Verification items for the finished model (mm, model axes). A direction names the side the tool comes from. Round coordinates to 2 decimals unless told otherwise and drop trailing zeros. Order: outer loops, then holes, each group sorted by start corner. A loop starts at its lowest first (then second) coordinate and runs counter-clockwise, first axis right, second up. Notation, with made-up numbers: (-11, 87) -> (34, 87) arc R8 cw to (34, 98) -> close; hole circle Ø9 at (-14.5, 79.5). An arc over 180 degrees is marked (long way). Return JSON: item names as keys, results as strings. Group by question number.
1) Section check C-C on x = -30. Enter the section's corners in (y, z), plus the area to 3 significant figures.
2) Depth check by flat-ended pin: pin 1 (5.5 mm diameter, centred on y = -22.6, z = -110.5, fed in from -X); pin 2 (4 mm diameter, centred on y = -20.5, z = -120, fed in from -X); pin 3 (0.6 mm diameter, centred on y = -1.5, z = -167.5, fed in from -X); pin 4 (1.6 mm diameter, centred on y = -1, z = -167.5, fed in from +X). Enter the tip coordinate at first touch or a pass-through.
3) Section check B-B on z = -148.5. Enter the section's corners in (x, y), plus the area to 3 significant figures.
4) Section check A-A on z = -34.5. Enter the section's corners in (x, y).
5) Scan lines: L1, parallel to Y at x = -18, z = -66; L2, parallel to X at y = -1, z = -34. Record each from-to range of solid material in increasing order.
6) Tool access check on faces 4 (the flat face through (-11, -1, -177.8)), 5 (the flat face through (-2, -17.9, -87.7)), 6 (the cylindrical face through (-27.1, -1, -72.4)), 7 (the cylindrical face through (-1, -22.5, -160)). Record the directions out of +Z, -Z, +X, -X, +Y, -Y that give a thin tool (end or side, any length) a straight path to the whole face; none if there is none.
7) Draft check along X on faces 1 (the cylindrical face through (-27.1, -1, -148.4)), 2 (the flat face through (0, -17, -88)), 3 (the cylindrical face through (-1, -22.7, -175)). Enter one of: pulls with the +X half, pulls with the -X half, needs draft (parallel to the pull), parting line crosses it, or undercut.
```python
from build123d import *

# Parameters (mm, degrees)
STRUCTURAL_MEMBER1_DEPTH        = 177.8
SLOT_DEPTH                      = 187.62491795
SKETCH4_R                       = 4.5
HOLE_DEPTH                      = 187.62491795
VERT_SLOT_DEPTH                 = 187.62491795
SLOT_PATTERN_COUNT              = 5
SLOT_PATTERN_PITCH              = 38
HOLE_PATTERN_COUNT              = 2
HOLE_PATTERN_PITCH              = 76
LPATTERN1_COUNT                 = 2
LPATTERN1_PITCH                 = 76
OTHER_SIDE_CUTS_COUNT           = 2
OTHER_SIDE_CUTS_ANGLE           = 90
OTHER_SIDE_CUTS_COPY_1_DEPTH    = 187.62491795
OTHER_SIDE_CUTS_COPY_2_DEPTH    = 187.62491795
OTHER_SIDE_CUTS_COPY_3_DEPTH    = 187.62491795
OTHER_SIDE_CUTS_COPY_4_DEPTH    = 187.62491795
OTHER_SIDE_CUTS_COPY_5_SKETCH_R = 4.5
OTHER_SIDE_CUTS_COPY_5_DEPTH    = 187.62491795
OTHER_SIDE_CUTS_COPY_6_DEPTH    = 187.62491795


with BuildPart() as part:
    # Sketch13 → Structural Member1 (new body)
    with BuildSketch(Plane(origin=(0, 0, 0), x_dir=(-1, 0, 0), z_dir=(0, 0, -1))):
        with BuildLine():
            Line((40.1, 0), (2, 0))
            ThreePointArc((2, 0), (0.585786438, -0.585786438), (0, -2))
            Line((0, -2), (0, -40.1))
            Line((0, -40.1), (1, -40.1))
            ThreePointArc((1, -40.1), (1.707106781, -39.807106781), (2, -39.1))
            Line((2, -39.1), (2, -4))
            ThreePointArc((2, -4), (2.585786438, -2.585786438), (4, -2))
            Line((4, -2), (39.1, -2))
            ThreePointArc((39.1, -2), (39.807106781, -1.707106781), (40.1, -1))
            Line((40.1, -1), (40.1, 0))
        make_face()
    extrude(amount=STRUCTURAL_MEMBER1_DEPTH)

    # Sketch3 → Slot (cut, through all)
    with BuildSketch(Plane(origin=(0, 0, 0), x_dir=(1, 0, 0), z_dir=(0, 1, 0))):
        with BuildLine():
            Line((-27.1, 12.5), (-27.1, 18.5))
            ThreePointArc((-27.1, 18.5), (-22.6, 23), (-18.1, 18.5))
            Line((-18.1, 18.5), (-18.1, 12.5))
            ThreePointArc((-18.1, 12.5), (-22.6, 8), (-27.1, 12.5))
        make_face()
    slot = extrude(amount=-SLOT_DEPTH, mode=Mode.SUBTRACT)

    # Sketch4 → Hole (cut, through all)
    with BuildSketch(Plane(origin=(0, 0, 0), x_dir=(1, 0, 0), z_dir=(0, 1, 0))):
        with Locations(Location((-22.6, 34.5, 0), (0, 0, 180))):
            Circle(SKETCH4_R)
    hole = extrude(amount=-HOLE_DEPTH, mode=Mode.SUBTRACT)

    # Sketch14 → Vert Slot (cut, through all)
    with BuildSketch(Plane(origin=(0, 0, 0), x_dir=(1, 0, 0), z_dir=(0, 1, 0))):
        with BuildLine():
            Line((-19.6, 68), (-22.6, 68))
            ThreePointArc((-22.6, 68), (-27.1, 72.5), (-22.6, 77))
            Line((-22.6, 77), (-19.6, 77))
            ThreePointArc((-19.6, 77), (-15.1, 72.5), (-19.6, 68))
        make_face()
    vert_slot = extrude(amount=-VERT_SLOT_DEPTH, mode=Mode.SUBTRACT)

    # Slot Pattern: Slot ×5
    with Locations(*[(0, 0, -i * SLOT_PATTERN_PITCH) for i in range(1, SLOT_PATTERN_COUNT)]):
        add(slot, mode=Mode.SUBTRACT)

    # Hole Pattern: Hole ×2
    with Locations(*[(0, 0, -i * HOLE_PATTERN_PITCH) for i in range(1, HOLE_PATTERN_COUNT)]):
        add(hole, mode=Mode.SUBTRACT)

    # LPattern1: Vert Slot ×2
    with Locations(*[(0, 0, -i * LPATTERN1_PITCH) for i in range(1, LPATTERN1_COUNT)]):
        add(vert_slot, mode=Mode.SUBTRACT)

    # Other side cuts: Slot, Hole, Vert Slot ×2 about axis
    other_side_cuts_axis = Axis((-4, -4, 0), (0, 0, 1))
    add([slot.rotate(other_side_cuts_axis, i * OTHER_SIDE_CUTS_ANGLE / (OTHER_SIDE_CUTS_COUNT - 1)) for i in range(1, OTHER_SIDE_CUTS_COUNT)], mode=Mode.SUBTRACT)
    add([hole.rotate(other_side_cuts_axis, i * OTHER_SIDE_CUTS_ANGLE / (OTHER_SIDE_CUTS_COUNT - 1)) for i in range(1, OTHER_SIDE_CUTS_COUNT)], mode=Mode.SUBTRACT)
    add([vert_slot.rotate(other_side_cuts_axis, i * OTHER_SIDE_CUTS_ANGLE / (OTHER_SIDE_CUTS_COUNT - 1)) for i in range(1, OTHER_SIDE_CUTS_COUNT)], mode=Mode.SUBTRACT)

    # Other side cuts copy 1 sketch → Other side cuts copy 1 (cut, through all)
    with BuildSketch(Plane(origin=(-8, 0, -38), x_dir=(0, 1, 0), z_dir=(-1, 0, 0))):
        with BuildLine():
            Line((-27.1, 12.5), (-27.1, 18.5))
            ThreePointArc((-27.1, 18.5), (-22.6, 23), (-18.1, 18.5))
            Line((-18.1, 18.5), (-18.1, 12.5))
            ThreePointArc((-18.1, 12.5), (-22.6, 8), (-27.1, 12.5))
        make_face()
    extrude(amount=-OTHER_SIDE_CUTS_COPY_1_DEPTH, mode=Mode.SUBTRACT)

    # Other side cuts copy 2 sketch → Other side cuts copy 2 (cut, through all)
    with BuildSketch(Plane(origin=(-8, 0, -76), x_dir=(0, 1, 0), z_dir=(-1, 0, 0))):
        with BuildLine():
            Line((-27.1, 12.5), (-27.1, 18.5))
            ThreePointArc((-27.1, 18.5), (-22.6, 23), (-18.1, 18.5))
            Line((-18.1, 18.5), (-18.1, 12.5))
            ThreePointArc((-18.1, 12.5), (-22.6, 8), (-27.1, 12.5))
        make_face()
    extrude(amount=-OTHER_SIDE_CUTS_COPY_2_DEPTH, mode=Mode.SUBTRACT)

    # Other side cuts copy 3 sketch → Other side cuts copy 3 (cut, through all)
    with BuildSketch(Plane(origin=(-8, 0, -114), x_dir=(0, 1, 0), z_dir=(-1, 0, 0))):
        with BuildLine():
            Line((-27.1, 12.5), (-27.1, 18.5))
            ThreePointArc((-27.1, 18.5), (-22.6, 23), (-18.1, 18.5))
            Line((-18.1, 18.5), (-18.1, 12.5))
            ThreePointArc((-18.1, 12.5), (-22.6, 8), (-27.1, 12.5))
        make_face()
    extrude(amount=-OTHER_SIDE_CUTS_COPY_3_DEPTH, mode=Mode.SUBTRACT)

    # Other side cuts copy 4 sketch → Other side cuts copy 4 (cut, through all)
    with BuildSketch(Plane(origin=(-8, 0, -152), x_dir=(0, 1, 0), z_dir=(-1, 0, 0))):
        with BuildLine():
            Line((-27.1, 12.5), (-27.1, 18.5))
            ThreePointArc((-27.1, 18.5), (-22.6, 23), (-18.1, 18.5))
            Line((-18.1, 18.5), (-18.1, 12.5))
            ThreePointArc((-18.1, 12.5), (-22.6, 8), (-27.1, 12.5))
        make_face()
    extrude(amount=-OTHER_SIDE_CUTS_COPY_4_DEPTH, mode=Mode.SUBTRACT)

    # Other side cuts copy 5 sketch → Other side cuts copy 5 (cut, through all)
    with BuildSketch(Plane(origin=(-8, 0, -76), x_dir=(0, 1, 0), z_dir=(-1, 0, 0))):
        with Locations(Location((-22.6, 34.5, 0), (0, 0, 180))):
            Circle(OTHER_SIDE_CUTS_COPY_5_SKETCH_R)
    extrude(amount=-OTHER_SIDE_CUTS_COPY_5_DEPTH, mode=Mode.SUBTRACT)

    # Other side cuts copy 6 sketch → Other side cuts copy 6 (cut, through all)
    with BuildSketch(Plane(origin=(-8, 0, -76), x_dir=(0, 1, 0), z_dir=(-1, 0, 0))):
        with BuildLine():
            Line((-19.6, 68), (-22.6, 68))
            ThreePointArc((-22.6, 68), (-27.1, 72.5), (-22.6, 77))
            Line((-22.6, 77), (-19.6, 77))
            ThreePointArc((-19.6, 77), (-15.1, 72.5), (-19.6, 68))
        make_face()
    extrude(amount=-OTHER_SIDE_CUTS_COPY_6_DEPTH, mode=Mode.SUBTRACT)


solid = part.part
```
Check result:
{
 "1": {"outline": "(-2, -177.8) -> (0, -177.8) -> (0, 0) -> (-2, 0) -> close", "area": "356 mm^2"},
 "2": {"pin 1": "through", "pin 2": "x = -2", "pin 3": "x = -40.08", "pin 4": "x = -0.01"},
 "3": {"outline": "(-40.1, -1) arc R1 ccw to (-39.1, -2) -> (-27.1, -2) -> (-27.1, 0) -> (-40.1, 0) -> close; (-15.1, -2) -> (-4, -2) arc R2 cw to (-2, -4) -> (-2, -15.1) -> (0, -15.1) -> (0, -2) arc R2 ccw to (-2, 0) -> (-15.1, 0) -> close; (-2, -39.1) arc R1 ccw to (-1, -40.1) -> (0, -40.1) -> (0, -27.1) -> (-2, -27.1) -> close", "area": "108 mm^2"},
 "4": {"outline": "(-40.1, -1) arc R1 ccw to (-39.1, -2) -> (-27.1, -2) -> (-27.1, 0) -> (-40.1, 0) -> close; (-18.1, -2) -> (-4, -2) arc R2 cw to (-2, -4) -> (-2, -18.1) -> (0, -18.1) -> (0, -2) arc R2 ccw to (-2, 0) -> (-18.1, 0) -> close; (-2, -39.1) arc R1 ccw to (-1, -40.1) -> (0, -40.1) -> (0, -27.1) -> (-2, -27.1) -> close"},
 "5": {"L1": "-2 to 0", "L2": "-40.1 to -27.07, -18.13 to -0.27"},
 "6": {"face 4": "-Z, +X, -X, +Y, -Y", "face 5": "+Z, -Z, -X, -Y", "face 6": "+Y, -Y", "face 7": "+X, -X"},
 "7": {"face 1": "undercut", "face 2": "pulls with the +X half", "face 3": "needs draft"}
}
